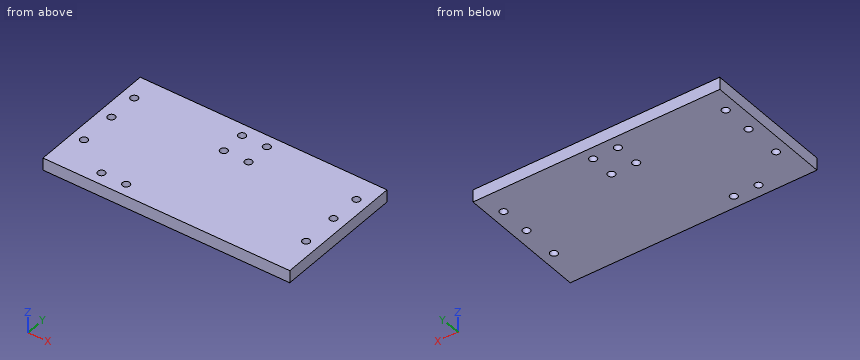
from build123d import *

# Parameters (mm, degrees)
SKETCH1_W           = 100
SKETCH1_H           = 53.16
BOSS_EXTRUDE1_DEPTH = 5
SKETCH2_R           = 1.5
CUT_EXTRUDE1_DEPTH  = 57.846252295


with BuildPart() as part:
    # Sketch1 → Boss-Extrude1 (new body)
    with BuildSketch(Plane.XY):
        Rectangle(SKETCH1_W, SKETCH1_H)
    extrude(amount=BOSS_EXTRUDE1_DEPTH)

    # Sketch2 → Cut-Extrude1 (cut, through all)
    with BuildSketch(Plane.XY.offset(5)):
        with Locations((-45, 16.58)):
            Circle(SKETCH2_R)
        with Locations((-45, 4.08)):
            Circle(SKETCH2_R)
        with Locations((-45, -10.92)):
            Circle(SKETCH2_R)
        with Locations(Location((45, -10.92, 0), (0, 0, 180))):
            Circle(SKETCH2_R)
        with Locations(Location((45, 4.08, 0), (0, 0, 180))):
            Circle(SKETCH2_R)
        with Locations(Location((45, 16.58, 0), (0, 0, 180))):
            Circle(SKETCH2_R)
        with Locations((-5, 11.58)):
            Circle(SKETCH2_R)
        with Locations((-5, 21.58)):
            Circle(SKETCH2_R)
        with Locations(Location((5, 11.58, 0), (0, 0, 180))):
            Circle(SKETCH2_R)
        with Locations(Location((5, 21.58, 0), (0, 0, 180))):
            Circle(SKETCH2_R)
        with Locations((-30, -21.58)):
            Circle(SKETCH2_R)
        with Locations((-20, -21.58)):
            Circle(SKETCH2_R)
    extrude(amount=-CUT_EXTRUDE1_DEPTH, mode=Mode.SUBTRACT)


solid = part.part
Source: CAD feature listing. Evaluate the final solid. Frame: model axes, mm. Round coordinates to 2 decimals unless told otherwise and drop trailing zeros. Order: outer loops, then holes, each group sorted by start corner. A loop starts at its lowest first (then second) coordinate and runs counter-clockwise, first axis right, second up. Notation, with made-up numbers: (8.25, -15.75) -> (42.25, -15.75) arc R26 ccw to (42.25, 9.25) -> close; hole circle Ø9 at (40, 12.5). An arc over 180 degrees is marked (long way). Answer as CSV lines item,"result".
Item 1: Line query: L1, parallel to Y at x = 5, z = 3.6; L2, parallel to X at y = -21.5, z = 4.1; L3, parallel to Y at x = 4, z = 2.6. Output: solid intervals per line, ascending.
A:
L1,"-26.58 to 10.08, 13.08 to 20.08, 23.08 to 26.58"
L2,"-50 to -31.5, -28.5 to -21.5, -18.5 to 50"
L3,"-26.58 to 10.46, 12.7 to 20.46, 22.7 to 26.58"
Item 2: Section C-C, the plane x = 45. Return loops of the section in (y, z).
A:
outline,"(-26.58, 0) -> (-12.42, 0) -> (-12.42, 5) -> (-26.58, 5) -> close; (-9.42, 0) -> (2.58, 0) -> (2.58, 5) -> (-9.42, 5) -> close; (5.58, 0) -> (15.08, 0) -> (15.08, 5) -> (5.58, 5) -> close; (18.08, 0) -> (26.58, 0) -> (26.58, 5) -> (18.08, 5) -> close"
Item 3: Section B-B, the plane y = 4.08. Return loops of the section in (x, z).
A:
outline,"(-50, 0) -> (-46.5, 0) -> (-46.5, 5) -> (-50, 5) -> close; (-43.5, 0) -> (43.5, 0) -> (43.5, 5) -> (-43.5, 5) -> close; (46.5, 0) -> (50, 0) -> (50, 5) -> (46.5, 5) -> close"
Item 4: Section A-A, the plane x = -20. Return loops of the section in (y, z).
A:
outline,"(-26.58, 0) -> (-23.08, 0) -> (-23.08, 5) -> (-26.58, 5) -> close; (-20.08, 0) -> (26.58, 0) -> (26.58, 5) -> (-20.08, 5) -> close"
Item 5: Section D-D, the plane z = 2.9. Count the separate pieces of the cut face and the enclosed holes in it, plus the area to 3 significant figures.
A:
separate pieces,"1"
enclosed holes,"12"
area,"5,230 mm²"
